```python
from build123d import *

# Parameters (mm, degrees)
F1_DEPTH = 4
F2_D     = 8
F3_D     = 3.5
F4_D     = 8
F5_D     = 3.5
F6_D     = 4.5
F7_D     = 3.5


with BuildPart() as f1:
    # F0 (on Top) → F1 (new body)
    with BuildSketch(Plane.XY):
        Polygon((-40, 90), (-66, 90), (-66, 70), (-41.2157141343, 70), (-40, 70), (-40, 62.8748962879), (-40, 56), (-40, 48), (-40, 0), (-66, 0), (-66, -120), (-40, -120), (-40, -128), (-40, -135.5958282948), (-40, -142), (-40, -190), (-66, -190), (-66, -230), (0, -230), (0, 56), (0, 62.8748962879), (0, 90), align=None)
        Polygon((66, 90), (0, 90), (0, 62.8748962879), (0, 56), (0, -230), (66, -230), (66, -190), (40, -190), (40, -142), (40, -128), (40, -120), (66, -120), (66, 0), (40, 0), (40, 48), (40, 70), (66, 70), align=None)
        with BuildLine():
            Line((0, 104), (0, 90))
            Line((0, 90), (66, 90))
            ThreePointArc((66, 90), (60.1421356237, 104.1421356237), (46, 110))
            Line((46, 110), (40, 110))
            Line((40, 110), (0, 110))
            Line((0, 110), (0, 104))
        make_face()
        Polygon((-40, 110), (-40, 90), (0, 90), (0, 104), (0, 110), (-6.6373916343, 110), align=None)
        with BuildLine():
            ThreePointArc((-46, 110), (-60.1421356237, 104.1421356237), (-66, 90))
            Line((-66, 90), (-40, 90))
            Line((-40, 90), (-40, 110))
            Line((-40, 110), (-46, 110))
        make_face()
    extrude(amount=F1_DEPTH)

    # F2 (through all)
    with Locations(Plane(origin=(0, 0, 0), x_dir=(1, 0, 0), z_dir=(0, 0, -1))):
        with Locations((-28, 128)):
            Hole(F2_D / 2)

    # F3 (through all)
    with Locations(Plane(origin=(0, 0, 0), x_dir=(1, 0, 0), z_dir=(0, 0, -1))):
        with Locations((-28, 142), (28, 142)):
            Hole(F3_D / 2)

    # F4 (through all)
    with Locations(Plane(origin=(0, 0, 0), x_dir=(1, 0, 0), z_dir=(0, 0, -1))):
        with Locations((28, 128)):
            Hole(F4_D / 2)

    # F5 (through all)
    with Locations(Plane(origin=(0, 0, 0), x_dir=(1, 0, 0), z_dir=(0, 0, -1))):
        with Locations((-28, -48), (28, -48)):
            Hole(F5_D / 2)

    # F6 (through all)
    with Locations(Plane(origin=(0, 0, 0), x_dir=(1, 0, 0), z_dir=(0, 0, -1))):
        with Locations((0, -56)):
            Hole(F6_D / 2)

    # F7 (through all)
    with Locations(Plane(origin=(0, 0, 0), x_dir=(1, 0, 0), z_dir=(0, 0, -1))):
        with Locations((0, -104)):
            Hole(F7_D / 2)


solid = f1.part
```
Design review of the part built by this model. Coordinates are the model's own, in mm. Coordinates: 2 decimals unless noted, no trailing zeros. Loops run counter-clockwise (first coordinate to the right, second up) from the corner with the lowest first, then second, coordinate; pieces in that order, holes last. Notation, with made-up numbers: (47.25, 7.5) - (97.25, 7.5) arc R27 ccw to (97.25, 23.5) - close; hole circle Ø7 at (62.25, -4). An arc over 180 degrees is marked (long way). Use CSV: the item, a comma, the result in double quotes. Start each with the question number.
1) Consider section B-B on x = -57. Write out the cut boundary in (y, z).
2) Consider section A-A on z = 2.6. Give the number of separate pieces and of enclosed holes in the cut face, then the cut area to 3 significant figures.
3) The part is to be moulded in two halves that separate along X. For faces 1 (the flat face through (-1, -58, 0)), 2 (the cylindrical face through (-59.986, 104.297, 1.972)), 3 (the cylindrical face through (-27.479, -131.966, 2.028)), 4 (the cylindrical face through (60.297, 103.986, 1.972)), say which applies: +X half, -X half, draft (parallel to the pull), parting line (faces both ways), or undercut.
4) Consider section C-C on y = 62. Write out the cut boundary in (x, z), then the cut area to 3 significant figures.
5) For pin 1 Ø2 at (x, z) = (-58.5, 2) entering from +Y; pin 2 Ø2 at (y, z) = (19, 2.5) entering from -X; pin 3 Ø2 at (x, z) = (57, 2.5) entering from +Y, all flat-tipped, find the tip position at first contact; note any pin that passes through.
6) Wall thickness on L1, parallel to X at y = -128, z = 3.05; L2, parallel to Y at x = -28, z = 1.8; L3, parallel to Y at x = -45.5, z = 1.3: over which ranges is each line inside the solid? List them lowest first. Write a range as from..to.
Geometry says:
1,outline,"(-230, 0) - (-190, 0) - (-190, 4) - (-230, 4) - close; (-120, 0) - (0, 0) - (0, 4) - (-120, 4) - close; (70, 0) - (106.7, 0) - (106.7, 4) - (70, 4) - close"
2,separate pieces,"1"
2,enclosed holes,"8"
2,area,"37,300 mm^2"
3,face 1,"draft"
3,face 2,"-X half"
3,face 3,"undercut"
3,face 4,"+X half"
4,outline,"(-40, 0) - (40, 0) - (40, 4) - (-40, 4) - close"
4,area,"320 mm^2"
5,pin 1,"y = 106.36"
5,pin 2,"x = -40"
5,pin 3,"y = 107.32"
6,L1,"-40..-32, -24..24, 32..40"
6,L2,"-230..-143.75, -140.25..-132, -124..46.25, 49.75..110"
6,L3,"-230..-190, -120..0, 70..110"
